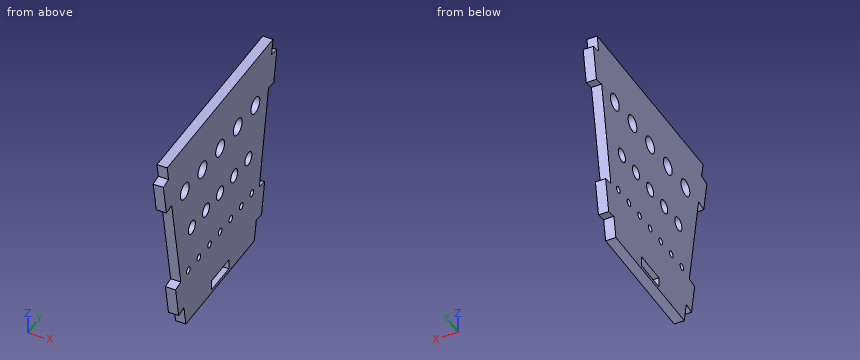
```python
from build123d import *

# Parameters (mm, degrees)
F0_W     = 10
F0_H     = 3
F0_R     = 1
F0_R_2   = 2
F0_R_3   = 2.5
F1_DEPTH = 3


with BuildPart() as f1:
    # F0 (on Right) → F1 (new body)
    with BuildSketch(Plane.YZ):
        Polygon((-20.527813, 6.280557), (-19.420381, 0), (19.420381, 0), (20.527813, 6.280557), (23.482236, 5.759612), (25.218718, 15.60769), (22.264295, 16.128634), (27.47374, 45.672867), (30.428163, 45.151922), (32.164645, 55), (29.210222, 55.520945), (30, 60), (-30, 60), (-29.210222, 55.520945), (-32.164645, 55), (-30.428163, 45.151922), (-27.47374, 45.672867), (-22.264295, 16.128634), (-25.218718, 15.60769), (-23.482236, 5.759612), align=None)
        with Locations((0, 2.5)):
            Rectangle(F0_W, F0_H, mode=Mode.SUBTRACT)
        with Locations((-18, 17)):
            Circle(F0_R, mode=Mode.SUBTRACT)
        with Locations((-12, 17)):
            Circle(F0_R, mode=Mode.SUBTRACT)
        with Locations((-6, 17)):
            Circle(F0_R, mode=Mode.SUBTRACT)
        with Locations((0, 17)):
            Circle(F0_R, mode=Mode.SUBTRACT)
        with Locations((6, 17)):
            Circle(F0_R, mode=Mode.SUBTRACT)
        with Locations((12, 17)):
            Circle(F0_R, mode=Mode.SUBTRACT)
        with Locations((18, 17)):
            Circle(F0_R, mode=Mode.SUBTRACT)
        with Locations((-16, 30)):
            Circle(F0_R_2, mode=Mode.SUBTRACT)
        with Locations((-8, 30)):
            Circle(F0_R_2, mode=Mode.SUBTRACT)
        with Locations((0, 30)):
            Circle(F0_R_2, mode=Mode.SUBTRACT)
        with Locations((-20, 45)):
            Circle(F0_R_3, mode=Mode.SUBTRACT)
        with Locations((-10, 45)):
            Circle(F0_R_3, mode=Mode.SUBTRACT)
        with Locations((0, 45)):
            Circle(F0_R_3, mode=Mode.SUBTRACT)
        with Locations((8, 30)):
            Circle(F0_R_2, mode=Mode.SUBTRACT)
        with Locations((16, 30)):
            Circle(F0_R_2, mode=Mode.SUBTRACT)
        with Locations((10, 45)):
            Circle(F0_R_3, mode=Mode.SUBTRACT)
        with Locations((20, 45)):
            Circle(F0_R_3, mode=Mode.SUBTRACT)
    extrude(amount=F1_DEPTH)


solid = f1.part
```
For this review, take the finished solid that the model builds, in its own axes (mm). Round coordinates to 2 decimals unless told otherwise and drop trailing zeros. Loops run counter-clockwise (first coordinate to the right, second up) from the corner with the lowest first, then second, coordinate; pieces in that order, holes last.
(1) We need section B-B (y = 0). Give the boundary of the cut face in (x, z).
Returned:
outline: (0, 0) - (3, 0) - (3, 1) - (0, 1) - close; (0, 4) - (3, 4) - (3, 16) - (0, 16) - close; (0, 18) - (3, 18) - (3, 28) - (0, 28) - close; (0, 32) - (3, 32) - (3, 42.5) - (0, 42.5) - close; (0, 47.5) - (3, 47.5) - (3, 60) - (0, 60) - close
(2) We need section C-C (z = 30). Give the boundary of the cut face in (x, y), plus the area to 3 significant figures.
Returned:
outline: (0, -24.71) - (3, -24.71) - (3, -18) - (0, -18) - close; (0, -14) - (3, -14) - (3, -10) - (0, -10) - close; (0, -6) - (3, -6) - (3, -2) - (0, -2) - close; (0, 2) - (3, 2) - (3, 6) - (0, 6) - close; (0, 10) - (3, 10) - (3, 14) - (0, 14) - close; (0, 18) - (3, 18) - (3, 24.71) - (0, 24.71) - close
area: 88.3 mm2
(3) Wall thickness on line 1 along Z through (x, y) = (1.15, 0); line 2 along Y through (x, z) = (1.15, 30.5); line 3 along Z through (x, y) = (1.25, -8): over which ranges is each line inside the solid? List them lowest first.
Returned:
line 1: z = 0 to 1, 4 to 16, 18 to 28, 32 to 42.5, 47.5 to 60
line 2: y = -24.8 to -17.94, -14.06 to -9.94, -6.06 to -1.94, 1.94 to 6.06, 9.94 to 14.06, 17.94 to 24.8
line 3: z = 0 to 28, 32 to 43.5, 46.5 to 60
(4) Clearance check with a flat-ended pin moving along its axis: P1, Ø0.9, axis at x = 1.5, z = 2.5, coming from the -Y side. State where the tip first meets the part, or that it passes through.
Returned:
P1: stops at y = -19.94
(5) We need section A-A (y = -16). Give the boundary of the cut face in (x, z), plus the area to 3 significant figures.
Returned:
outline: (0, 0) - (3, 0) - (3, 28) - (0, 28) - close; (0, 32) - (3, 32) - (3, 60) - (0, 60) - close
area: 168 mm2
(6) We need section D-D (x = 2.35). State how many separate pieces and enclosed holes the cut face has, plus the area to 3 significant figures.
Returned:
separate pieces: 1
enclosed holes: 18
area: 2,870 mm2
